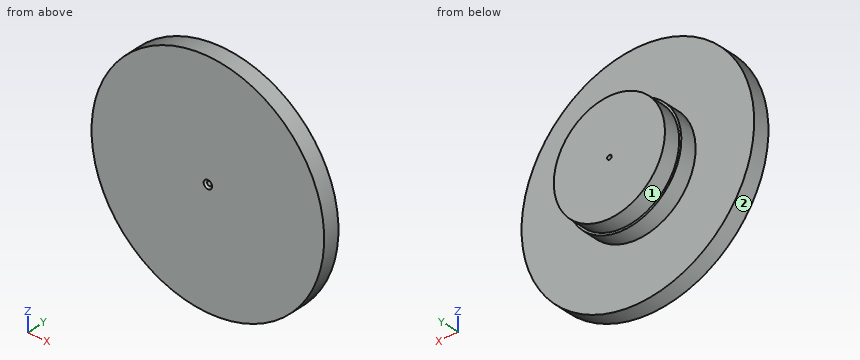
```python
from build123d import *

# Parameters (mm, degrees)
SKETCH1_R                                           = 84.9884
BOSS_EXTRUDE1_DEPTH                                 = 76.2
SKETCH1_3_R                                         = 88.265
SKETCH1_3_R_2                                       = 84.9884
BOSS_EXTRUDE2_DEPTH                                 = 50.8
SKETCH1_4_R                                         = 177.8
SKETCH1_4_R_2                                       = 88.265
BOSS_EXTRUDE3_DEPTH                                 = 25.4
CSK_FOR_1_4_FLAT_HEAD_MACHINE_SCREW_100_D           = 6.7564
CSK_FOR_1_4_FLAT_HEAD_MACHINE_SCREW_100_CSINK_D     = 12.8778
CSK_FOR_1_4_FLAT_HEAD_MACHINE_SCREW_100_CSINK_ANGLE = 100


with BuildPart() as part:
    # Sketch1 → Boss-Extrude1 (new body)
    with BuildSketch(Plane(origin=(0, 0, 0), x_dir=(1, 0, 0), z_dir=(0, 1, 0))):
        with Locations(Location((0, 0, 0), (0, 0, 90))):
            Circle(SKETCH1_R)
    extrude(amount=BOSS_EXTRUDE1_DEPTH)

    # Sketch1_3 → Boss-Extrude2 (add)
    with BuildSketch(Plane(origin=(0, 0, 0), x_dir=(1, 0, 0), z_dir=(0, 1, 0))):
        with Locations(Location((0, 0, 0), (0, 0, 270))):
            Circle(SKETCH1_3_R)
        with Locations(Location((0, 0, 0), (0, 0, 90))):
            Circle(SKETCH1_3_R_2, mode=Mode.SUBTRACT)
    extrude(amount=BOSS_EXTRUDE2_DEPTH)

    # Sketch1_4 → Boss-Extrude3 (add)
    with BuildSketch(Plane(origin=(0, 0, 0), x_dir=(1, 0, 0), z_dir=(0, 1, 0))):
        with Locations(Location((0, 0, 0), (0, 0, 270))):
            Circle(SKETCH1_4_R)
        with Locations(Location((0, 0, 0), (0, 0, 270))):
            Circle(SKETCH1_4_R_2, mode=Mode.SUBTRACT)
    extrude(amount=BOSS_EXTRUDE3_DEPTH)

    # CSK for 1_4 Flat Head Machine Screw _100 (through all)
    with Locations(Plane(origin=(0, 0, 0), x_dir=(-1, 0, 0), z_dir=(0, -1, 0))):
        with Locations((0, 0)):
            CounterSinkHole(CSK_FOR_1_4_FLAT_HEAD_MACHINE_SCREW_100_D / 2, CSK_FOR_1_4_FLAT_HEAD_MACHINE_SCREW_100_CSINK_D / 2, counter_sink_angle=CSK_FOR_1_4_FLAT_HEAD_MACHINE_SCREW_100_CSINK_ANGLE)


solid = part.part
```
CAD build for the part. Positions are in the model's coordinates, mm. Face numbers are marked on the shaded views. A direction names the side the tool comes from. Round coordinates to 2 decimals unless told otherwise and drop trailing zeros. Loops run counter-clockwise (first coordinate to the right, second up) from the corner with the lowest first, then second, coordinate; pieces in that order, holes last. Notation, with made-up numbers: (66.25, 7) - (110.25, 7) arc R27 ccw to (110.25, 33) - close; hole circle Ø10 at (-10, 52). An arc over 180 degrees is marked (long way). Return JSON: item names as keys, results as strings. Group by question number.
Q1. Drill centre lines: line 1 along Y through (x, z) = (90, -73.5); line 2 along Z through (x, y) = (-66, 35.5); line 3 along X through (y, z) = (51, 76). Where is each one in solid material? Low to high. Write a range as [from, to].
Q2. Band-saw the part on A-A on y = 37. Give the cut face in (x, z) (3 decimals), plus the area to 3 significant figures.
Q3. Flat gauge pins, fed straight in: pin 1 Ø1.5 at (x, z) = (-104.5, -86) entering from +Y; pin 2 Ø10 at (x, y) = (25, 47.5) entering from +Z; pin 3 Ø3 at (x, y) = (-131, 26.5) entering from -Z. Where does each tip first touch, or does it go through?
Q4. Band-saw the part on D-D on x = 134. Give the cut face in (y, z), plus the area to 3 significant figures.
Q5. Band-saw the part on B-B on x = -28.5. Give the cut face in (y, z).
Q6. Band-saw the part on C-C on z = -62.5. Give the cut face in (x, y), plus the area to 3 significant figures.
Q7. Tool access for the marked faces 1 and 2: list every direction of +Z, -Z, +X, -X, +Y, -Y with a clear straight run to the whole face (end or side of a thin tool).
Solutions:
{
 "1": {"line 1": "y = [0, 25.4]", "line 2": "z = [-58.61, 58.61]", "line 3": "x = [-38.04, 38.04]"},
 "2": {"outline": "circle Ø176.53 at (0, 0); hole circle Ø6.756 at (0, 0)", "area": "24,400 mm^2"},
 "3": {"pin 1": "stops at y = 25.4", "pin 2": "stops at z = 85.97", "pin 3": "stops at z = -121.32"},
 "4": {"outline": "(0, -116.86) - (25.4, -116.86) - (25.4, 116.86) - (0, 116.86) - close", "area": "5,940 mm^2"},
 "5": {"outline": "(0, -175.5) - (25.4, -175.5) - (25.4, -83.54) - (50.8, -83.54) - (50.8, -80.07) - (76.2, -80.07) - (76.2, 80.07) - (50.8, 80.07) - (50.8, 83.54) - (25.4, 83.54) - (25.4, 175.5) - (0, 175.5) - close"},
 "6": {"outline": "(-166.45, 0) - (166.45, 0) - (166.45, 25.4) - (62.33, 25.4) - (62.33, 50.8) - (57.59, 50.8) - (57.59, 76.2) - (-57.59, 76.2) - (-57.59, 50.8) - (-62.33, 50.8) - (-62.33, 25.4) - (-166.45, 25.4) - close", "area": "14,500 mm^2"},
 "7": {"face 1": "+Y", "face 2": "+Y, -Y"}
}
